from build123d import *

# Parameters (mm, degrees)
ESQUISSE1_R             = 5
BASE_EXTRUSION_DEPTH    = 6
ESQUISSE2_R             = 6
BOSS_EXTRU_1_DEPTH      = 60
ESQUISSE3_R             = 4
BOSS_EXTRU_2_DEPTH      = 6
CHANFREIN1_SIZE         = 0.5
ESQUISSE4_R             = 2.5
ENL_V_MAT_EXTRU_1_DEPTH = 7


with BuildPart() as part:
    # Esquisse1 → Base-Extrusion (new body)
    with BuildSketch(Plane.XY):
        with Locations(Location((0, 0, 0), (0, 0, 180))):
            Circle(ESQUISSE1_R)
    extrude(amount=BASE_EXTRUSION_DEPTH)

    # Esquisse2 → Boss.-Extru.1 (add)
    with BuildSketch(Plane.XY.offset(6)):
        with Locations(Location((0, 0, 0), (0, 0, 180))):
            Circle(ESQUISSE2_R)
    extrude(amount=BOSS_EXTRU_1_DEPTH)

    # Esquisse3 → Boss.-Extru.2 (add)
    with BuildSketch(Plane.XY.offset(66)):
        with Locations(Location((0, 0, 0), (0, 0, 180))):
            Circle(ESQUISSE3_R)
    extrude(amount=BOSS_EXTRU_2_DEPTH)

    # Chanfrein1
    chanfrein1_edges = [part.edges().sort_by_distance(p)[0] for p in [
        (6, 0, 6),
        (6, 0, 66),
        (5, 0, 0),
        (4, 0, 72),
    ]]
    chamfer(chanfrein1_edges, length=CHANFREIN1_SIZE)

    # Esquisse4 → Enlèv. mat.-Extru.1 (cut)
    with BuildSketch(Plane(origin=(0, 0, 0), x_dir=(1, 0, 0), z_dir=(0, 1, 0))):
        with Locations(Location((0, -44, 0), (0, 0, 270))):
            Circle(ESQUISSE4_R)
    extrude(amount=-ENL_V_MAT_EXTRU_1_DEPTH, mode=Mode.SUBTRACT)


solid = part.part
CAD build for the part. Positions are in the model's coordinates, mm. A direction names the side the tool comes from. Coordinates: 2 decimals unless noted, no trailing zeros. Loops run counter-clockwise (first coordinate to the right, second up) from the corner with the lowest first, then second, coordinate; pieces in that order, holes last. Notation, with made-up numbers: (50, -11) -> (65, -11) arc R35 cw to (65, 21) -> close; hole circle Ø10 at (-15.5, 46.25). An arc over 180 degrees is marked (long way). One line per item, written item: value.
1. Which spindle directions (+Z, -Z, +X, -X, +Y, -Y) get a long thin tool onto all of the face, cutting with end or side? Do faces 5 (the face through (0.1, -3, 41.5)), 6 (the face through (4, 2, 66)), 7 (the face through (0, 0, 0)), 8 (the face through (5, 0, 3)). Say none if no direction does.
Answers:
face 5: -Y
face 6: +Z
face 7: -Z, +X, -X, +Y, -Y
face 8: -Z
2. Drill centre lines: line 1 (Z direction, x = 0, y = -1.75); line 2 (Z direction, x = 0, y = -4.5); line 3 (X direction, y = -1.25, z = 44). Where is each one in solid material? Low to high. Write a range as [from, to].
Answers:
line 1: z = [0, 41.5], [46.5, 72]
line 2: z = [0, 41.5], [46.5, 66]
line 3: x = [-5.87, -2.5], [2.5, 5.87]
3. Slice it at B-B on z = 5. Write the cut outline in (x, y).
Answers:
outline: circle Ø10 at (0, 0)
4. Pull direction Z, two halves, no side cores. Call faces 1 (the face through (-2.769, 5.323, 35.587)), 2 (the face through (-1.6, 4.9, 6)), 3 (the face through (0, 0, 44)), 4 (the face through (0, 0, 72)): pulls with the +Z half, pulls with the -Z half, needs draft (parallel to the pull), parting line crosses it, or undercut.
Answers:
face 1: needs draft
face 2: pulls with the -Z half
face 3: undercut
face 4: pulls with the +Z half
5. Slice it at A-A on x = 0. Write the cut outline in (y, z).
Answers:
outline: (-6, 6.5) -> (-5.5, 6) -> (-5, 6) -> (-5, 0.5) -> (-4.5, 0) -> (4.5, 0) -> (5, 0.5) -> (5, 6) -> (5.5, 6) -> (6, 6.5) -> (6, 65.5) -> (5.5, 66) -> (4, 66) -> (4, 71.5) -> (3.5, 72) -> (-3.5, 72) -> (-4, 71.5) -> (-4, 66) -> (-5.5, 66) -> (-6, 65.5) -> (-6, 46.5) -> (0, 46.5) -> (0, 41.5) -> (-6, 41.5) -> close
6. Flat gauge pins, fed straight in: P1, Ø6, axis at x = -5, y = -1.5, coming from the -Z side; P2, Ø3, axis at x = -3.5, z = 17.5, coming from the -Y side; P3, Ø3, axis at y = 4, z = 14, coming from the +X side; P4, Ø1, axis at y = -1, z = 43, coming from the -X side. Where does each tip first touch, or does it go through?
Answers:
P1: stops at z = 0
P2: stops at y = -5.66
P3: stops at x = 5.45
P4: stops at x = -5.98
7. Slice it at D-D on z = 44. Write the cut outline in (x, y), and give its area (3 significant figures).
Answers:
outline: (-2.5, -5.45) -> (-2.5, 0) -> (2.5, 0) -> (2.5, -5.45) arc R6 ccw (long way) to start
area: 84.0 mm^2
8. Slice it at C-C on z = 25. Write the cut outline in (x, y), and give its area (3 significant figures).
Answers:
outline: circle Ø12 at (0, 0)
area: 113 mm^2
